from build123d import *

# Parameters (mm, degrees)
SKETCH2_R           = 1.5
BOSS_EXTRUDE1_DEPTH = 18
SKETCH3_W           = 10
SKETCH3_H           = 12
CUT_EXTRUDE1_DEPTH  = 32
SKETCH4_W           = 27
SKETCH4_H           = 5
BOSS_EXTRUDE3_DEPTH = 12
SKETCH8_R           = 1.5
CUT_EXTRUDE3_DEPTH  = 12
FILLET1_R           = 3
FILLET2_R           = 3
FILLET3_R           = 3
FILLET4_R           = 3


with BuildPart() as part:
    # Sketch2 → Boss-Extrude1 (new body)
    with BuildSketch(Plane.XY):
        Polygon((0, 0), (27, 0), (27, -12), (27, -16), (0, -16), (0, -12), align=None)
        with Locations((4.5, -6)):
            Circle(SKETCH2_R, mode=Mode.SUBTRACT)
        with Locations((22.5, -6)):
            Circle(SKETCH2_R, mode=Mode.SUBTRACT)
    extrude(amount=BOSS_EXTRUDE1_DEPTH)

    # Sketch3 → Cut-Extrude1 (cut)
    with BuildSketch(Plane.ZY):
        with Locations((9, -6)):
            Rectangle(SKETCH3_W, SKETCH3_H)
    extrude(amount=-CUT_EXTRUDE1_DEPTH, mode=Mode.SUBTRACT)

    # Sketch4 → Boss-Extrude3 (add)
    with BuildSketch(Plane.XZ.offset(16)):
        with Locations((13.5, 11.947290181)):
            Rectangle(SKETCH4_W, SKETCH4_H)
        with Locations((13.5, 6.947290181)):
            Rectangle(SKETCH4_W, SKETCH4_H)
    extrude(amount=BOSS_EXTRUDE3_DEPTH)

    # Sketch8 → Cut-Extrude3 (cut)
    with BuildSketch(Plane(origin=(0, 0, 4.447290181), x_dir=(-1, 0, 0), z_dir=(0, 0, -1))):
        with Locations((-13.5, -23.5)):
            Circle(SKETCH8_R)
        with BuildLine():
            Line((-27, -21.451026779), (-27, -28))
            Line((-27, -28), (0, -28))
            Line((0, -28), (0, -21.451026779))
            ThreePointArc((0, -21.451026779), (-13.5, -27.996407915), (-27, -21.451026779))
        make_face()
    extrude(amount=-CUT_EXTRUDE3_DEPTH, mode=Mode.SUBTRACT)

    # Fillet1
    fillet1_edges = [part.edges().sort_by_distance(p)[0] for p in [
        (0, 0, 2),
    ]]
    fillet(fillet1_edges, radius=FILLET1_R)

    # Fillet2
    fillet2_edges = [part.edges().sort_by_distance(p)[0] for p in [
        (27, 0, 2),
    ]]
    fillet(fillet2_edges, radius=FILLET2_R)

    # Fillet3
    fillet3_edges = [part.edges().sort_by_distance(p)[0] for p in [
        (0, 0, 16),
    ]]
    fillet(fillet3_edges, radius=FILLET3_R)

    # Fillet4
    fillet4_edges = [part.edges().sort_by_distance(p)[0] for p in [
        (27, 0, 16),
    ]]
    fillet(fillet4_edges, radius=FILLET4_R)


solid = part.part
Check sheet for the modelled part. Datum: model origin and axes. Units: mm. A direction names the side the tool comes from. Coordinates: 2 decimals unless noted, no trailing zeros. Write each loop counter-clockwise with the first axis right and the second up, starting at its lowest first coordinate (ties: lowest second). Pieces come first, ordered by that corner, then holes. Notation, with made-up numbers: M 60,-32 L 69,-32 A24 ccw 69,-8 Z; hole C 80.25,-29 d6. An arc over 180 degrees is marked long. Answer as CSV lines item,"result".
Q1. Set-up check for faces 5 (the face through (27, -12.4, 8.9)), 6 (the face through (14, -16, 2)), 7 (the face through (13.283, -27.995, 9.377)), 8 (the face through (13, -12, 9)), 9 (the face through (13, -21, 14.447)): record each of +Z, -Z, +X, -X, +Y, -Y from which the full face is reachable in a straight line by a thin tool's end or side.
Check result:
face 5,"+Z, -Z, +X, +Y, -Y"
face 6,"-Z, +X, -X, -Y"
face 7,"+Z, -Z, -Y"
face 8,"+X, -X, +Y"
face 9,"+Z, +X, -X, -Y"
Q2. Material ranges on probe 1 along X at (y, z) = (-6, 16.95); probe 2 along Y at (x, z) = (4.5, 15.85); probe 3 along Z at (x, y) = (24.5, -6.5), recorded low to high. Write a range as from..to.
Check result:
probe 1,"0..3, 6..21, 24..27"
probe 2,"-16..-7.5, -4.5..0"
probe 3,"0..4, 14..18"
Q3. Mould release check, pull along X, two halves, no side actions. Record for faces 1 (the face through (26.1, -0.86, 16.03)), 2 (the face through (0.9, -0.86, 2.03)), 3 (the face through (13, -21, 4.447)), 4 (the face through (14.61, -22.49, 9.38)): released by +X, released by -X, zero draft, split by the parting line, or undercut.
Check result:
face 1,"released by +X"
face 2,"released by -X"
face 3,"zero draft"
face 4,"undercut"
Q4. Cross-section at D-D (y = -9). Record the boundary of the cut face in (x, z), then the cut area to 3 significant figures.
Check result:
outline,"M 0,0 L 27,0 L 27,4 L 0,4 Z; M 0,14 L 27,14 L 27,18 L 0,18 Z"
area,"216 mm^2"
Q5. Go/stop test with flat-tipped pins: pin 1 (1.5 mm diameter, centred on x = 5.5, z = 13, fed in from -Y); pin 2 (1.8 mm diameter, centred on x = 4.5, y = -6, fed in from -Z); pin 3 (1.3 mm diameter, centred on x = 17.5, z = 3, fed in from -Y); pin 4 (2 mm diameter, centred on x = 11, z = 12.5, fed in from -Y). Record where each tip stops, or that it passes through.
Check result:
pin 1,"y = -26.39"
pin 2,"through"
pin 3,"y = -16"
pin 4,"y = -27.93"
Q6. Cross-section at B-B (y = -6). Record the boundary of the cut face in (x, z).
Check result:
outline,"M 0,0 L 3,0 L 3,4 L 0,4 Z; M 0,14 L 3,14 L 3,18 L 0,18 Z; M 6,0 L 21,0 L 21,4 L 6,4 Z; M 6,14 L 21,14 L 21,18 L 6,18 Z; M 24,0 L 27,0 L 27,4 L 24,4 Z; M 24,14 L 27,14 L 27,18 L 24,18 Z"
Q7. Cross-section at C-C (x = 13.5). Record the boundary of the cut face in (y, z).
Check result:
outline,"M -28,4.45 L -25,4.45 L -25,14.45 L -28,14.45 Z; M -22,4.45 L -16,4.45 L -16,0 L 0,0 L 0,4 L -12,4 L -12,14 L 0,14 L 0,18 L -16,18 L -16,14.45 L -22,14.45 Z"
Q8. Cross-section at A-A (z = 15.25). Record the boundary of the cut face in (x, y).
Check result:
outline,"M 0,-16 L 27,-16 L 27,-3 A3 ccw 24,0 L 3,0 A3 ccw 0,-3 Z; hole C 4.5,-6 d3; hole C 22.5,-6 d3"
